```python
from build123d import *

# Parameters (mm, degrees)
F1_DEPTH = 11.90625


# Not quite as in the source:
# - a length typed as a fraction of an inch, garbled in the dataset ("3 / 203.2 mm" for 3/8 in), is restored


with BuildPart() as f1:
    # F0 (on Top) → F1 (new body)
    with BuildSketch(Plane.XY):
        with BuildLine():
            ThreePointArc((0, 9.1178910807), (-5.1898410508, 9.6890057882), (-10.2093555033, 8.2519613206))
            Line((-10.2093555033, 8.2519613206), (-12.369341217, 7.1464567445))
            Line((-12.369341217, 7.1464567445), (-12.369341217, 4.6386048198))
            Line((-12.369341217, 4.6386048198), (-12.369341217, 4.5682978211))
            ThreePointArc((-12.369341217, 4.5682978211), (-15.5930977879, 3.1185654947), (-17.7027139134, 0.2823972963))
            ThreePointArc((-17.7027139134, 0.2823972963), (-18.3641606661, -4.889059653), (-17.5542831421, -10.0393583998))
            ThreePointArc((-17.5542831421, -10.0393583998), (-13.4613837791, -13.3941238354), (-8.5996589687, -15.484556372))
            ThreePointArc((-8.5996589687, -15.484556372), (-5.0294162563, -15.0523544446), (-2.1409380715, -12.9098966718))
            Line((-2.1409380715, -12.9098966718), (0, -14.2561570176))
            Line((0, -14.2561570176), (1.9696742658, -12.9098966718))
            ThreePointArc((1.9696742658, -12.9098966718), (4.9392756736, -15.0084468105), (8.560301624, -15.3410370587))
            ThreePointArc((8.560301624, -15.3410370587), (13.367982191, -13.3015402533), (17.4874793738, -10.0916987285))
            ThreePointArc((17.4874793738, -10.0916987285), (18.16772005, -4.8427956267), (17.6633565687, 0.4259166096))
            ThreePointArc((17.6633565687, 0.4259166096), (15.4847616458, 3.3168082822), (12.1560195839, 4.739132713))
            Line((12.1560195839, 4.739132713), (12.1560195839, 7.1464567445))
            Line((12.1560195839, 7.1464567445), (9.9960338703, 8.2519613206))
            ThreePointArc((9.9960338703, 8.2519613206), (5.0827762692, 9.6633625741), (0, 9.1178910807))
        make_face()
    extrude(amount=F1_DEPTH)


solid = f1.part
```
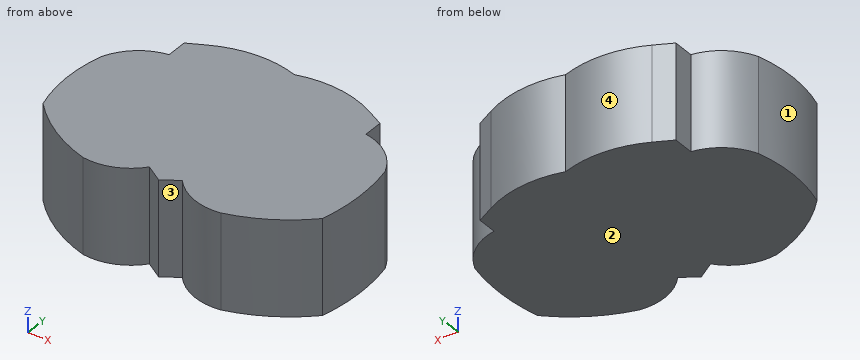
Geometry check sheet. Reference: the model listing, model coordinates, mm. Face numbers are marked on the shaded views. Round coordinates to 2 decimals unless told otherwise and drop trailing zeros. Order: outer loops, then holes, each group sorted by start corner. A loop starts at its lowest first (then second) coordinate and runs counter-clockwise, first axis right, second up. Notation, with made-up numbers: (80.5, -26) - (121.5, -26) arc R31 ccw to (121.5, 1) - close; hole circle Ø2 at (-4, 67.5). An arc over 180 degrees is marked (long way). Use a Markdown table: item, result. Add a question column.
(1) Material ranges on line 1 along X through (y, z) = (-4.25, 8.75); line 2 along X through (y, z) = (6.5, 2.75); line 3 along X through (y, z) = (-13.75, 5.5), recorded low to high. Write a range as [from, to].
(2) Depth check by flat-ended pin: pin 1 (5 mm diameter, centred on y = -2, z = 10.5, fed in from -X); pin 2 (1.5 mm diameter, centred on y = 3, z = 8.5, fed in from +X); pin 3 (1 mm diameter, centred on x = 14, z = 5.5, fed in from -Y); pin 4 (3 mm diameter, centred on x = -6, z = 7, fed in from +Y). Enter the tip coordinate at first touch or a pass-through.
(3) Sectioned sample at A-A, the plane z = 2. Enter the section's corners in (x, y).
(4) Sectioned sample at C-C, the plane y = 2.75. Enter the section's corners in (x, z), and give its area (3 significant figures).
(5) Release check for a two-part mould opening along X. For the marked faces 1, 2, 3 and 4 record: pulls with the +X half, pulls with the -X half, needs draft (parallel to the pull), parting line crosses it, or undercut.
(6) Sectioned sample at B-B, the plane x = -8. Enter the section's corners in (y, z), and give its area (3 significant figures).
Answers below:
| question | item | result |
|---|---|---|
| 1 | line 1 | [-18.36, 18.17] |
| 1 | line 2 | [-12.37, 12.16] |
| 1 | line 3 | [-12.85, -2.93], [-0.8, 0.74], [2.8, 12.56] |
| 2 | pin 1 | x = -18.37 |
| 2 | pin 2 | x = 16.58 |
| 2 | pin 3 | y = -13.22 |
| 2 | pin 4 | y = 9.73 |
| 3 | outline | (-17.7, 0.28) arc R18.47 ccw to (-17.55, -10.04) arc R18.93 ccw to (-8.6, -15.48) arc R7.02 ccw to (-2.14, -12.91) - (0, -14.26) - (1.97, -12.91) arc R7.02 ccw to (8.56, -15.34) arc R20.09 ccw to (17.49, -10.09) arc R23.64 ccw to (17.66, 0.43) arc R7.02 ccw to (12.16, 4.74) - (12.16, 7.15) - (10, 8.25) arc R13.3 ccw to (0, 9.12) arc R13.53 ccw to (-10.21, 8.25) - (-12.37, 7.15) - (-12.37, 4.57) arc R7.02 ccw to start |
| 4 | outline | (-16.02, 0) - (16.12, 0) - (16.12, 11.91) - (-16.02, 11.91) - close |
| 4 | area | 383 mm² |
| 5 | face 1 | pulls with the -X half |
| 5 | face 2 | needs draft |
| 5 | face 3 | undercut |
| 5 | face 4 | undercut |
| 6 | outline | (-15.54, 0) - (9.15, 0) - (9.15, 11.91) - (-15.54, 11.91) - close |
| 6 | area | 294 mm² |
